```python
from build123d import *

# Parameters (mm, degrees)
F1_DEPTH = 25.4
F2_R     = 42.08433
F3_DEPTH = 25.4
F5_DEPTH = 50.8


with BuildPart() as f1:
    # F0 (on Top) → F1 (new body)
    with BuildSketch(Plane.XY):
        Polygon((-3.173529, 76.703862), (-68.014258, 35.603574), (-64.840729, -41.100288), (3.173529, -76.703862), (68.014258, -35.603574), (64.840729, 41.100288), align=None)
    extrude(amount=F1_DEPTH)

    # F2 (on face) → F3 (join)
    with BuildSketch(Plane.XY.offset(25.4)):
        Circle(F2_R)
    extrude(amount=F3_DEPTH)

    # F4 (on face) → F5 (cut, through all)
    with BuildSketch(Plane.XY.offset(50.8)):
        Polygon((3.518755, 24.523791), (-19.478848, 15.309226), (-22.997603, -9.214564), (-3.518755, -24.523791), (19.478848, -15.309226), (22.997603, 9.214564), align=None)
    extrude(amount=-F5_DEPTH, mode=Mode.SUBTRACT)


solid = f1.part
```
Check sheet for the modelled part. Datum: model origin and axes. Units: mm. A direction names the side the tool comes from. Give positions to 0.01 mm unless a question says otherwise; leave off trailing zeros. Order: outer loops, then holes, each group sorted by start corner. A loop starts at its lowest first (then second) coordinate and runs counter-clockwise, first axis right, second up. Notation, with made-up numbers: M 41.5,-12.75 L 87.5,-12.75 A34 cw 87.5,23.25 Z; hole C -11.5,26 d2. An arc over 180 degrees is marked long. Answer in a Markdown table with one row per item.
1) Cross-section at A-A, the plane x = 0. Enter the section's corners in (y, z), plus the area to 3 significant figures.
Filled sheet:
| item | result |
|---|---|
| outline | M -75.04,0 L -23.11,0 L -23.11,50.8 L -42.08,50.8 L -42.08,25.4 L -75.04,25.4 Z; M 23.11,0 L 75.04,0 L 75.04,25.4 L 42.08,25.4 L 42.08,50.8 L 23.11,50.8 Z |
| area | 3,600 mm2 |
2) Access from +Z, -Z, +X, -X, +Y, -Y to the whole of each face (thin tool, end or side, straight path). Record for faces 1 (the flat face through (-9.941, 19.293, 50.8)), 2 (the cylindrical face through (40.14, 12.64, 37.92)), 3 (the flat face through (-7.82, 19.98, 25.76)).
Filled sheet:
| item | result |
|---|---|
| face 1 | +Z, +X, -X, +Y, -Y |
| face 2 | +Z |
| face 3 | +Z, -Z |
3) Cross-section at C-C, the plane z = 16. Enter the section's corners in (x, y).
Filled sheet:
| item | result |
|---|---|
| outline | M -68.01,35.6 L -64.84,-41.1 L 3.17,-76.7 L 68.01,-35.6 L 64.84,41.1 L -3.17,76.7 Z; hole M -23,-9.21 L -3.52,-24.52 L 19.48,-15.31 L 23,9.21 L 3.52,24.52 L -19.48,15.31 Z |
4) Cross-section at B-B, the plane y = -13. Enter the section's corners in (x, z).
Filled sheet:
| item | result |
|---|---|
| outline | M -66,0 L -18.18,0 L -18.18,50.8 L -40.03,50.8 L -40.03,25.4 L -66,25.4 Z; M 19.81,0 L 67.08,0 L 67.08,25.4 L 40.03,25.4 L 40.03,50.8 L 19.81,50.8 Z |
5) Cross-section at D-D, the plane x = -36. Enter the section's corners in (y, z).
Filled sheet:
| item | result |
|---|---|
| outline | M -56.2,0 L 55.9,0 L 55.9,25.4 L 21.8,25.4 L 21.8,50.8 L -21.8,50.8 L -21.8,25.4 L -56.2,25.4 Z |
6) Gauge pin test, flat ends, axial feed: P1, Ø3, axis at x = 34, z = 40, coming from the +Y side; P2, Ø8, axis at x = 38, y = -44, coming from the +Z side; P3, Ø5, axis at x = -4.5, z = 36, coming from the -Y side. Record the tip position at first contact, or that the pin passes through.
Filled sheet:
| item | result |
|---|---|
| P1 | stops at y = 26.74 |
| P2 | stops at z = 25.4 |
| P3 | stops at y = -42.04 |
7) Thickness scan on L1, parallel to Z at x = 50, y = -45; L2, parallel to Y at x = 5, z = 4; L3, parallel to Y at x = 19, z = 37. Record the ranges inside material, lowest first. Write a range as [from, to].
Filled sheet:
| item | result |
|---|---|
| L1 | z = [0, 25.4] |
| L2 | y = [-75.55, -21.11], [23.36, 72.43] |
| L3 | y = [-37.55, -15.5], [12.36, 37.55] |
8) Release check for a two-part mould opening along X. For faces 4 (the flat face through (-35.14, 56.44, 12.52)), 5 (the flat face through (21.214, -3.219, 25.756)), 6 (the flat face through (31.31, 58.653, 12.522)) record: +X half, -X half, draft (parallel to the pull), parting line (faces both ways), or undercut.
Filled sheet:
| item | result |
|---|---|
| face 4 | -X half |
| face 5 | undercut |
| face 6 | +X half |
